Source: CAD feature listing. Evaluate the final solid. Frame: model axes, mm. A direction names the side the tool comes from. Coordinates: 2 decimals unless noted, no trailing zeros. Order: outer loops, then holes, each group sorted by start corner. A loop starts at its lowest first (then second) coordinate and runs counter-clockwise, first axis right, second up.
```python
from build123d import *

# Parameters (mm, degrees)
F1_DEPTH    = 44.45
F2_W        = 30
F2_H        = 25.4
F3_DEPTH    = 88.9
F4_T4_DEPTH = 216.4
F4_S6_R     = 19.05
F4_T7_DEPTH = 111
F5_R        = 9.525
F6_DEPTH    = 12.7
F7_R        = 2
F8_DEPTH    = 5
F9_R        = 9.525
F10_DEPTH   = 24.5
F11_R       = 7
F12_DEPTH   = 7.5


# Not quite as in the source:
# - a fillet or chamfer that OpenCascade refuses, or shapes differently, is made with other operations: its cross-section is extruded or revolved along the edge and cut away or added


with BuildPart() as f1:
    # F0 (on Front) → F1 (new body)
    with BuildSketch(Plane.XZ):
        with BuildLine():
            Line((0, 0), (19.05, 0))
            ThreePointArc((19.05, 0), (0, 19.05), (-19.05, 0))
            Line((-19.05, 0), (0, 0))
        make_face()
        with BuildLine():
            Line((44.45, 0), (19.05, 0))
            ThreePointArc((19.05, 0), (0, -19.05), (-19.05, 0))
            Line((-19.05, 0), (-44.45, 0))
            Line((-44.45, 0), (-44.45, -25.4))
            Line((-44.45, -25.4), (-15.875, -25.4))
            Line((-15.875, -25.4), (-15.875, -44.45))
            Line((-15.875, -44.45), (-11.1125, -44.45))
            Line((-11.1125, -44.45), (-11.1125, -49.2125))
            Line((-11.1125, -49.2125), (-15.875, -49.2125))
            Line((-15.875, -49.2125), (-15.875, -69.85))
            Line((-15.875, -69.85), (15.875, -69.85))
            Line((15.875, -69.85), (15.875, -49.2125))
            Line((15.875, -49.2125), (11.1125, -49.2125))
            Line((11.1125, -49.2125), (11.1125, -44.45))
            Line((11.1125, -44.45), (15.875, -44.45))
            Line((15.875, -44.45), (15.875, -25.4))
            Line((15.875, -25.4), (44.45, -25.4))
            Line((44.45, -25.4), (44.45, 0))
        make_face()
        with BuildLine():
            ThreePointArc((-19.05, 0), (0, -19.05), (19.05, 0))
            Line((19.05, 0), (0, 0))
            Line((0, 0), (-19.05, 0))
        make_face()
    extrude(amount=F1_DEPTH)

    # F2 (on face) → F3 (join)
    with BuildSketch(Plane(origin=(-44.45, 0, 0), x_dir=(0, -1, 0), z_dir=(-1, 0, 0))):
        with Locations((15, 12.7)):
            Rectangle(F2_W, F2_H)
    extrude(amount=-F3_DEPTH)

    # F4: fillet of radius 25.5 on 1 edges, made by hand


with BuildPart() as f4_tool2:
    # F4_s3 → F4_t4 (new body)
    with BuildSketch(Plane.YZ.offset(-108.2)):
        with BuildLine():
            ThreePointArc((-30, -0.1), (-22.5312229203, 17.9312229203), (-4.5, 25.4))
            Line((-4.5, 25.4), (-30, 25.4))
            Line((-30, 25.4), (-30, -0.1))
        make_face()
    extrude(amount=F4_T4_DEPTH)

    split(bisect_by=Plane.XY, keep=Keep.TOP)

    # F4_s6 → F4_t7 (cut, symmetric)
    with BuildSketch(Plane.XZ.offset(17.2)):
        Circle(F4_S6_R)
    extrude(amount=F4_T7_DEPTH, both=True, mode=Mode.SUBTRACT)


with BuildPart() as f1_1:
    add(f1.part)

    # F4_t1: cut F4_tool2
    add(f4_tool2.part, mode=Mode.SUBTRACT)

    # F5 (on face) → F6 (cut)
    with BuildSketch(Plane.XZ.offset(44.45)):
        Circle(F5_R)
    extrude(amount=-F6_DEPTH, mode=Mode.SUBTRACT)

    # F7 (on face) → F8 (cut)
    with BuildSketch(Plane(origin=(0, 0, 0), x_dir=(-1, 0, 0), z_dir=(0, 1, 0))):
        with BuildLine():
            ThreePointArc((-27.45, 10.4), (-29.45, 12.4), (-31.45, 10.4))
            ThreePointArc((-31.45, 10.4), (-29.45, 8.4), (-27.45, 10.4))
        make_face()
        with Locations((29.45, 10.4)):
            Circle(F7_R)
    extrude(amount=-F8_DEPTH, mode=Mode.SUBTRACT)

    # F9 (on face) → F10 (join)
    with BuildSketch(Plane.XZ.offset(44.45)):
        Circle(F9_R)
    extrude(amount=-F10_DEPTH)

    # F11 (on face) → F12 (cut)
    with BuildSketch(Plane.XZ.offset(44.45)):
        Circle(F11_R)
    extrude(amount=-F12_DEPTH, mode=Mode.SUBTRACT)


solid = f1_1.part
```
1. Draft query along Z for faces 1 (the flat face through (-13, -22, -49.212)), 2 (the flat face through (-44.45, -17, -5)), 3 (the flat face through (30, -22, -25.4)). Return one class per face: +Z half, -Z half, draft (parallel to the pull), parting line (faces both ways), or undercut.
2. Contact query for flat-ended pins moving along their axis: P1, Ø4.5, axis at x = 29.5, z = 9.5, coming from the +Y side; P2, Ø1, axis at y = -5.5, z = -55, coming from the -X side (3 decimals); P3, Ø11.5, axis at x = 34, y = -36, coming from the +Z side; P4, Ø4, axis at y = -19, z = -46.5, coming from the +X side. Output: stop coordinate, or through.
3. Section query D-D, the plane x = 13. Output: boundary loops of the cut face in (y, z), plus the area to 3 significant figures.
4. Access query for faces 4 (the flat face through (-14, -22, -44.45)), 5 (the flat face through (-15.875, -22, -35)), 6 (the flat face through (-29, -5, 10)), 7 (the flat face through (15.875, -22, -35)), 8 (the flat face through (11.112, -22, -47)). Directions: +Z, -Z, +X, -X, +Y, -Y. A direction counts if a zero-diameter tool reaches every point of the face in a straight line with its end or side. Return the directions, or none.
5. Section query C-C, the plane z = 2. Output: boundary loops of the cut face in (x, y), plus the area to 3 significant figures.
6. Section query A-A, the plane x = 29.45. Output: boundary loops of the cut face in (y, z).
7. Material intervals for line 1 along Z through (x, y) = (-29.45, -3.65); line 2 along Z through (x, y) = (0, -39); line 3 along X through (y, z) = (-3, 9), sorted ascending.
Answer key:
1. face 1: undercut
1. face 2: draft
1. face 3: -Z half
2. P1: stops at y = 0
2. P2: stops at x = -15.875
2. P3: stops at z = 0
2. P4: stops at x = 11.11
3. outline: (-44.45, -69.85) - (0, -69.85) - (0, -49.21) - (-44.45, -49.21) - close; (-44.45, -44.45) - (0, -44.45) - (0, 25.4) - (-4.5, 25.4) arc R25.5 ccw to (-25.8, 13.92) - (-44.45, 13.92) - close
3. area: 3,740 mm2
4. face 4: -X, +Y, -Y
4. face 5: -Z, -X, +Y, -Y
4. face 6: +Y
4. face 7: -Z, +X, +Y, -Y
4. face 8: +X, +Y, -Y
5. outline: (-44.45, -29.91) - (-18.94, -29.91) - (-18.94, -44.45) - (-6.71, -44.45) - (-6.71, -36.95) - (6.71, -36.95) - (6.71, -44.45) - (18.94, -44.45) - (18.94, -29.91) - (44.45, -29.91) - (44.45, 0) - (-44.45, 0) - close
5. area: 3,110 mm2
6. outline: (-44.45, -25.4) - (0, -25.4) - (0, 8.4) - (-5, 8.4) - (-5, 12.4) - (0, 12.4) - (0, 25.4) - (-4.5, 25.4) arc R25.5 ccw to (-30, 0) - (-44.45, 0) - close
7. line 1: z = -25.4 to 8.4, 12.4 to 25.4
7. line 2: z = -69.85 to -7, 7 to 19.05
7. line 3: x = -44.45 to -30.88, -28.02 to 28.02, 30.88 to 44.45
